Work out the finished part from the listing and answer in its coordinate system (mm). Face numbers are marked on the shaded views. A direction names the side the tool comes from. Round coordinates to 2 decimals unless told otherwise and drop trailing zeros. Loops run counter-clockwise (first coordinate to the right, second up) from the corner with the lowest first, then second, coordinate; pieces in that order, holes last. Notation, with made-up numbers: M 84.5,56 L 138.5,56 A10 cw 138.5,61 Z; hole C 1,-33.5 d3. An arc over 180 degrees is marked long. One line per item, written item: value.
```python
from build123d import *

# Parameters (mm, degrees)
BOSS_EXTRUDE2_DEPTH = 4
BOSS_EXTRUDE4_DEPTH = 10.5
SKETCH9_R           = 3
CUT_EXTRUDE1_DEPTH  = 10


with BuildPart() as part:
    # Sketch1 → Boss-Extrude2 (new body)
    with BuildSketch(Plane(origin=(0, 0, 0), x_dir=(1, 0, 0), z_dir=(0, 1, 0))):
        Polygon((0, 0), (0, 25), (75, 25), (75, -25), (0, -25), align=None)
    extrude(amount=BOSS_EXTRUDE2_DEPTH)

    # Sketch7 → Boss-Extrude4 (add)
    with BuildSketch(Plane(origin=(0, 4, 0), x_dir=(1, 0, 0), z_dir=(0, 1, 0))):
        Polygon((0, 0), (0, 17), (34, 17), (34, -17), (0, -17), align=None)
    extrude(amount=BOSS_EXTRUDE4_DEPTH)

    # Sketch9 → Cut-Extrude1 (cut)
    with BuildSketch(Plane(origin=(0, 4, 0), x_dir=(1, 0, 0), z_dir=(0, 1, 0))):
        with Locations((69.078986276, 0)):
            Circle(SKETCH9_R)
    extrude(amount=-CUT_EXTRUDE1_DEPTH, mode=Mode.SUBTRACT)


solid = part.part
```
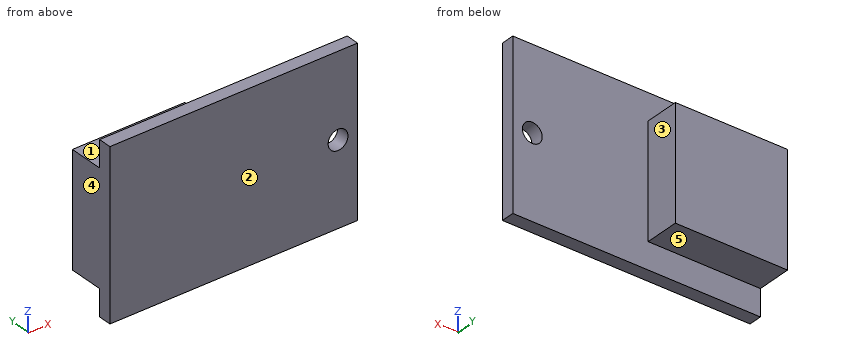
1) Find section D-D (y = 9.75). Give the vertices of the cut face in (x, z).
Check values:
outline: M 0,-17 L 34,-17 L 34,17 L 0,17 Z
2) Find section A-A (z = 0). Give the vertices of the cut face in (x, y).
Check values:
outline: M 0,0 L 66.08,0 L 66.08,4 L 34,4 L 34,14.5 L 0,14.5 Z; M 72.08,0 L 75,0 L 75,4 L 72.08,4 Z
3) Each of these flat-tipped pins is pushed along its axis until it touches: pin 1 (1 mm diameter, centred on x = 40, z = 17.5, fed in from -Y); pin 2 (5 mm diameter, centred on x = 67.5, z = 18, fed in from +Y); pin 3 (3 mm diameter, centred on x = 20, y = 7, fed in from +Z); pin 4 (5 mm diameter, centred on y = 9.5, z = -4, fed in from +X). Where does it stop, or does it pass through?
Check values:
pin 1: y = 0
pin 2: y = 4
pin 3: z = 17
pin 4: x = 34
4) Find section B-B (z = -5.5). Give the vertices of the cut face in (x, y).
Check values:
outline: M 0,0 L 75,0 L 75,4 L 34,4 L 34,14.5 L 0,14.5 Z
5) Find section C-C (x = 32.5). Give the vertices of the cut face in (y, z), then the cut area to 3 significant figures.
Check values:
outline: M 0,-25 L 4,-25 L 4,-17 L 14.5,-17 L 14.5,17 L 4,17 L 4,25 L 0,25 Z
area: 557 mm2
6) Find the intervals of material crossed by probe 1 along X at (y, z) = (1.4, 0); probe 2 along Y at (x, z) = (52, 12.5); probe 3 along X at (y, z) = (4.5, -12.5), in increasing order. Write a range as from..to.
Check values:
probe 1: 0..66.08, 72.08..75
probe 2: 0..4
probe 3: 0..34
7) For the marked faces 1, 2, 3, 4 and 5, determine the directions among +Z, -Z, +X, -X, +Y, -Y from which every point of the face is accessible in a straight line to the end or side of a thin tool.
Check values:
face 1: +Z, +X, -X, +Y
face 2: +Z, -Z, +X, -X, -Y
face 3: +Z, -Z, +X, +Y
face 4: +Z, -Z, -X, +Y, -Y
face 5: -Z, +X, -X, +Y
